For this review, take the finished solid that the model builds, in its own axes (mm). A direction names the side the tool comes from. Round coordinates to 2 decimals unless told otherwise and drop trailing zeros. Loops run counter-clockwise (first coordinate to the right, second up) from the corner with the lowest first, then second, coordinate; pieces in that order, holes last.
1. Tool access review of faces 5 (the cylindrical face through (10.974, 10.461, -0.076)), 6 (the cylindrical face through (0.225, 8.063, 6.735)), 7 (the flat face through (0, 6, -4.762)): name each direction out of +Z, -Z, +X, -X, +Y, -Y from which nothing blocks a thin tool from reaching the whole face with its end or side.
2. Draft analysis for pull direction Y (two halves, no side actions). For faces 1 (the flat face through (-4.144, 6.261, 2.348)), 2 (the flat face through (-5, 12.7, -2)), 3 (the cylindrical face through (-10.2, 6.3, -0.1)), 4 (the flat face through (-16, 3.85, 0)), state which applies: released by +Y, released by -Y, zero draft, split by the parting line, or undercut.
3. To check wall thickness, follow line 1 along X through (y, z) = (10.8, 0); line 2 along Z through (x, y) = (12.7, 11); line 3 along Y through (x, z) = (0, 7.35). State the ranges of each line that lie inside material, in increasing order.
4. Clearance check with flat-ended pins moving along their axes: pin 1 Ø1.9 at (x, z) = (-12, 0) entering from +Y; pin 2 Ø2 at (x, z) = (12.7, 0) entering from +Y; pin 3 Ø2 at (y, z) = (7.5, -3.5) entering from -X. State where each tip first meets the part, or that it passes through.
5. Consider section C-C on y = 9.25. State the section outline as (x, z) points.
6. Consider section A-A on x = 0. State the section outline as (y, z) points, then the cut area to 3 significant figures.
7. Consider section B-B on z = 5.25. State the section outline as (x, y) points.
8. Consider section D-D on z = 3. State the section outline as (x, y) points, then the cut area to 3 significant figures.
from build123d import *

# Parameters (mm, degrees)
SKETCH1_W                  = 38.1
SKETCH1_H                  = 17.526
BOSS_EXTRUDE1_DEPTH        = 12.7
CUT_EXTRUDE1_DEPTH         = 25.4
F_8_32_TAPPED_HOLE1_REACH  = 26.515
F_8_32_TAPPED_HOLE1_BORE_R = 1.7272
MIRROR1_START              = -8.763
MIRROR1_DEPTH              = 17.526
MIRROR1_START_2            = 8.85
MIRROR1_2_OUTLINE_R        = 1.7272
MIRROR1_2_DEPTH            = 5.15
F_8_32_TAPPED_HOLE2_D      = 3.4544
F_8_32_TAPPED_HOLE2_DEPTH  = 10.668
F_8_32_TAPPED_HOLE2_TIP    = 1.037806461


with BuildPart() as part:
    # Sketch1 → Boss-Extrude1 (new body)
    with BuildSketch(Plane(origin=(0, 0, 0), x_dir=(1, 0, 0), z_dir=(0, 1, 0))):
        Rectangle(SKETCH1_W, SKETCH1_H)
        Polygon((5.499261314, 0), (2.749630657, 4.7625), (-2.749630657, 4.7625), (-5.499261314, 0), (-2.749630657, -4.7625), (2.749630657, -4.7625), align=None, mode=Mode.SUBTRACT)
    extrude(amount=BOSS_EXTRUDE1_DEPTH)

    # Sketch2 → Cut-Extrude1 (cut)
    with BuildSketch(Plane.XY.offset(8.763)):
        with BuildLine():
            Line((12.7, 8.85), (19.05, 8.85))
            ThreePointArc((19.05, 8.85), (21.55, 6.35), (19.05, 3.85))
            Line((19.05, 3.85), (12.7, 3.85))
            ThreePointArc((12.7, 3.85), (10.2, 6.35), (12.7, 8.85))
        make_face()
    extrude(amount=-CUT_EXTRUDE1_DEPTH, mode=Mode.SUBTRACT)

    # #8-32 Tapped Hole1 bore → #8-32 Tapped Hole1 (cut, up to next)
    with BuildSketch(Plane(origin=(0, 12.7, 0), x_dir=(1, 0, 0), z_dir=(0, 1, 0)), mode=Mode.PRIVATE) as f_8_32_tapped_hole1_sk1:
        with Locations((12.7, 0)):
            Circle(F_8_32_TAPPED_HOLE1_BORE_R)
    f_8_32_tapped_hole1_tool1 = extrude(f_8_32_tapped_hole1_sk1.sketch, amount=-F_8_32_TAPPED_HOLE1_REACH, mode=Mode.PRIVATE) & part.part
    add(f_8_32_tapped_hole1_tool1.solids().sort_by_distance((12.7, 12.7, 0))[0], mode=Mode.SUBTRACT)

    # Mirror1: read off the stored shape, not the designer's step
    # Mirror1 outline → Mirror1 (cut)
    with BuildSketch(Plane.XY.offset(MIRROR1_START)):
        with BuildLine():
            Line((-12.7, 8.85), (-19.05, 8.85))
            Line((-19.05, 8.85), (-19.05, 3.85))
            Line((-19.05, 3.85), (-12.7, 3.85))
            ThreePointArc((-12.7, 3.85), (-10.2, 6.35), (-12.7, 8.85))
        make_face()
    extrude(amount=MIRROR1_DEPTH, mode=Mode.SUBTRACT)

    # Mirror1 2 outline → Mirror1 2 (cut)
    with BuildSketch(Plane(origin=(0, 0, 0), x_dir=(1, 0, 0), z_dir=(0, 1, 0)).offset(MIRROR1_START_2)):
        with Locations((-12.7, 0)):
            Circle(MIRROR1_2_OUTLINE_R)
    extrude(amount=MIRROR1_2_DEPTH, mode=Mode.SUBTRACT)

    # #8-32 Tapped Hole2
    with Locations(Plane.XY.offset(8.763)):
        with Locations((0, 6.35)):
            Hole(F_8_32_TAPPED_HOLE2_D / 2, depth=F_8_32_TAPPED_HOLE2_DEPTH)
            with Locations((0, 0, -(F_8_32_TAPPED_HOLE2_DEPTH + F_8_32_TAPPED_HOLE2_TIP / 2))):  # 118° drill point
                Cone(0, F_8_32_TAPPED_HOLE2_D / 2, F_8_32_TAPPED_HOLE2_TIP, mode=Mode.SUBTRACT)


solid = part.part
Resolved:
1. face 5: +Y
1. face 6: +Z
1. face 7: +Y, -Y
2. face 1: zero draft
2. face 2: released by +Y
2. face 3: undercut
2. face 4: undercut
3. line 1: x = -19.05 to -14.43, -10.97 to -5.5, 5.5 to 10.97, 14.43 to 19.05
3. line 2: z = -8.76 to -1.73, 1.73 to 8.76
3. line 3: y = 0 to 4.62, 8.08 to 12.7
4. pin 1: stops at y = 8.85
4. pin 2: stops at y = 4.06
4. pin 3: stops at x = -11.42
5. outline: (-19.05, -8.76) - (19.05, -8.76) - (19.05, 8.76) - (-19.05, 8.76) - close; hole circle Ø3.45 at (-12.7, 0); hole (-5.5, 0) - (-2.75, -4.76) - (2.75, -4.76) - (5.5, 0) - (2.75, 4.76) - (-2.75, 4.76) - close; hole circle Ø3.45 at (12.7, 0)
6. outline: (0, -8.76) - (12.7, -8.76) - (12.7, -4.76) - (0, -4.76) - close; (0, 4.76) - (4.62, 4.76) - (4.62, 8.76) - (0, 8.76) - close; (8.08, 4.76) - (12.7, 4.76) - (12.7, 8.76) - (8.08, 8.76) - close
6. area: 87.8 mm2
7. outline: (-19.05, 0) - (19.05, 0) - (19.05, 3.85) - (12.7, 3.85) arc R2.5 cw to (12.7, 8.85) - (19.05, 8.85) - (19.05, 12.7) - (-19.05, 12.7) - (-19.05, 8.85) - (-12.7, 8.85) arc R2.5 cw to (-12.7, 3.85) - (-19.05, 3.85) - close; hole circle Ø3.45 at (0, 6.35)
8. outline: (-19.05, 0) - (-3.77, 0) - (-3.77, 12.7) - (-19.05, 12.7) - (-19.05, 8.85) - (-12.7, 8.85) arc R2.5 cw to (-12.7, 3.85) - (-19.05, 3.85) - close; (3.77, 0) - (19.05, 0) - (19.05, 3.85) - (12.7, 3.85) arc R2.5 cw to (12.7, 8.85) - (19.05, 8.85) - (19.05, 12.7) - (3.77, 12.7) - close
8. area: 305 mm2
